Autodesk Inventor part; units mm, degrees
ref_plane "YZ Plane" through (0, 0, 0) normal (1, 0, 0) x (0, 1, 0)
ref_plane "XZ Plane" through (0, 0, 0) normal (0, 1, 0) x (-1, 0, 0)
ref_plane "XY Plane" through (0, 0, 0) normal (0, 0, 1) x (1, 0, 0)
sketch "Boceto1" plane through (0, 0, 0) normal (0, 0, 1) x (1, 0, 0)
  circle A0 centre (0, 0) radius 30
  circle A1 centre (0, 0) radius 26.15
  circle A2 centre (940, 0) radius 30
  circle A3 centre (940, 0) radius 26.15
  line L0 (22.3607, -20) -> (917.6393, -20)
  line L1 (26.15, 0) -> (30, 0)
  line L2 (910, 0) -> (940, 0)
  line L3 (22.3607, 20) -> (917.6393, 20)
  dimension "d1" = 52.3
  dimension "d0" = 60
  dimension "d2" = 940
  dimension "d3" = 60
  dimension "d4" = 52.3
extrude "Extrusión1" add sketch "Boceto1" along normal blind 80
sketch "Boceto2" plane through (0, 0, 80) normal (0, 0, 1) x (1, 0, 0)
  arc A0 (22.3607, 20) -> (22.3607, -20) centre (0, 0) ccw
  line L0 (22.3607, -20) -> (917.6393, -20)
  arc A1 (917.6393, -20) -> (917.6393, 20) centre (940, 0) ccw
  line L1 (917.6393, 20) -> (22.3607, 20)
  circle A2 centre (0, 0) radius 26.15
  circle A3 centre (940, 0) radius 26.15
  line L2 (917.6393, 20) -> (22.3607, 20)
  circle A4 centre (0, 0) radius 30
  circle A5 centre (940, 0) radius 30
  point P0 (22.3607, -20)
extrude "Extrusión2" add sketch "Boceto2" along normal blind 80 contours A4 A0 | A1 A5
properties part number "bocina1"
Check sheet for the modelled part. Datum: model origin and axes. Units: mm. A direction names the side the tool comes from. Give positions to 0.01 mm unless a question says otherwise; leave off trailing zeros. Order: outer loops, then holes, each group sorted by start corner. A loop starts at its lowest first (then second) coordinate and runs counter-clockwise, first axis right, second up. Notation, with made-up numbers: M 71,76 L 125,76 A28 ccw 125,112 Z; hole C 33,88 d4. An arc over 180 degrees is marked long. Answer in a Markdown table with one row per item.
1) Cross-section at C-C, the plane z = 149. Enter the section's corners in (x, y).
Filled sheet:
| item | result |
|---|---|
| outline | M 22.36,-20 A30 ccw 22.36,20 A30 ccw long Z; C 940,0 d60; hole C 0,0 d52.3; hole C 940,0 d52.3 |
2) Cross-section at B-B, the plane x = 0. Enter the section's corners in (y, z), plus the area to 3 significant figures.
Filled sheet:
| item | result |
|---|---|
| outline | M -30,0 L -26.15,0 L -26.15,160 L -30,160 Z; M 26.15,0 L 30,0 L 30,160 L 26.15,160 Z |
| area | 1,230 mm2 |
3) Thickness scan on L1, parallel to Y at x = 0, z = 38; L2, parallel to X at y = 19, z = 31.5; L3, parallel to X at y = -18.5, z = 20.5. Record the ranges inside material, lowest first. Write a range as [from, to].
Filled sheet:
| item | result |
|---|---|
| L1 | y = [-30, -26.15], [26.15, 30] |
| L2 | x = [-23.22, -17.97], [17.97, 922.03], [957.97, 963.22] |
| L3 | x = [-23.62, -18.48], [18.48, 921.52], [958.48, 963.62] |
4) Gauge pin test, flat ends, axial feed: P1, Ø10, axis at x = 644.5, z = 32, coming from the -Y side; P2, Ø5, axis at x = 709.5, y = -19.5, coming from the +Z side; P3, Ø1.5, axis at y = 14, z = 70.5, coming from the +X side. Record the tip position at first contact, or that the pin passes through.
Filled sheet:
| item | result |
|---|---|
| P1 | stops at y = -20 |
| P2 | stops at z = 80 |
| P3 | stops at x = 966.92 |
5) Release check for a two-part mould opening along X. For faces 1 (the cylindrical face through (-29.983, -1.013, 119.44)), 2 (the flat face through (463, 0, 0)) record: +X half, -X half, draft (parallel to the pull), parting line (faces both ways), or undercut.
Filled sheet:
| item | result |
|---|---|
| face 1 | undercut |
| face 2 | draft |
6) Access from +Z, -Z, +X, -X, +Y, -Y to the whole of each face (thin tool, end or side, straight path). Record for faces 3 (the cylindrical face through (30, 0, 119)), 4 (the flat face through (464, 20, 39)), 5 (the flat face through (464, 0, 80)), 6 (the flat face through (464, -20, 39)), 7 (the flat face through (-9, 25, 160)).
Filled sheet:
| item | result |
|---|---|
| face 3 | +Z |
| face 4 | +Z, -Z, +Y |
| face 5 | +Z, +Y, -Y |
| face 6 | +Z, -Z, -Y |
| face 7 | +Z, +X, -X, +Y, -Y |
7) Cross-section at A-A, the plane y = 0. Enter the section's corners in (x, z).
Filled sheet:
| item | result |
|---|---|
| outline | M -30,0 L -26.15,0 L -26.15,160 L -30,160 Z; M 26.15,0 L 913.85,0 L 913.85,160 L 910,160 L 910,80 L 30,80 L 30,160 L 26.15,160 Z; M 966.15,0 L 970,0 L 970,160 L 966.15,160 Z |
